The model under review builds one solid part; all positions refer to its coordinate system, in mm. A direction names the side the tool comes from. Give positions to 0.01 mm unless a question says otherwise; leave off trailing zeros. Order: outer loops, then holes, each group sorted by start corner. A loop starts at its lowest first (then second) coordinate and runs counter-clockwise, first axis right, second up. Notation, with made-up numbers: (79, 52) - (103, 52) arc R24 ccw to (103, 68) - close; hole circle Ø7 at (38.5, -29.75). An arc over 180 degrees is marked (long way). Write item = value, one per line. Start each with the question number.
1. Wall thickness on probe 1 along X at (y, z) = (62, 24) (3 decimals); probe 2 along X at (y, z) = (-233, 38.5); probe 3 along Y at (x, z) = (133, 7.5): over which ranges is each line inside the solid? List them lowest first.
2. Mouldability with a two-part tool opening along Y and no side actions: class faces 4 (the flat face through (322, 71.069, 70)), 5 (the flat face through (317.5, -165, 66)), 6 (the flat face through (176.452, 115.669, 10.908)) as pulls with the +Y half, pulls with the -Y half, needs draft (parallel to the pull), parting line crosses it, or undercut.
3. We need section B-B, the plane y = -259. Give the boundary of the cut face in (x, z) (3 decimals), and give its area (3 significant figures).
4. We need section C-C, the plane z = 73.5. Give the boundary of the cut face in (x, y) (3 decimals).
5. For P1, Ø7.5, axis at x = 320.5, z = 69, coming from the -Y side; P2, Ø6, axis at x = 322, z = 65.5, coming from the +Y side; P3, Ø6, axis at x = 162.5, z = 108.5, coming from the +Y side; P4, Ø3.5, axis at x = 147.5, y = 109, coming from the +Z side, all flat-tipped, find the tip position at first contact; note any pin that passes through.
6. We need section D-D, the plane y = -86. Give the boundary of the cut face in (x, z) (3 decimals), and give its area (3 significant figures).
7. We need section A-A, the plane x = 183. Give the boundary of the cut face in (y, z), and give its area (3 significant figures).
8. Machinability: for faces 1 (the flat face through (324, 74.244, 71)), 2 (the flat face through (0, -56, 50)), 3 (the flat face through (164.245, -284.866, 16.28)), which of the approach directions +Z, -Z, +X, -X, +Y, -Y give a long, thin tool a straight path to every point of the face, cutting with its end or side? Answer none if there is none.
from build123d import *

# Parameters (mm, degrees)
F1_DEPTH = 330
F2_T     = -3.175
F3_W     = 304.8
F3_H     = 101.6
F4_DEPTH = 254
F5_W     = 304.8
F5_H     = 254
F6_DEPTH = 25.4


with BuildPart() as f1:
    # F0 (on Right) → F1 (new body)
    with BuildSketch(Plane.YZ):
        Polygon((-18.4111015737, 126.7885861181), (-333.886384964, 0), (126.113615036, 0), (74.243833744, 54.1712634957), (74.243833744, 89.1712634957), align=None)
    extrude(amount=F1_DEPTH)

    # F2
    f2_openings = [f1.faces().sort_by_distance(p)[0] for p in [
        (165, -103.886385, 0),
    ]]
    offset(amount=F2_T, openings=f2_openings, kind=Kind.INTERSECTION)

    # F3 (on Front) → F4 (cut)
    with BuildSketch(Plane.XZ):
        with Locations((165.1896406174, 66.1754549101)):
            Rectangle(F3_W, F3_H)
    extrude(amount=-F4_DEPTH, mode=Mode.SUBTRACT)

    # F5 (on face) → F6 (cut)
    with BuildSketch(Plane(origin=(0, -46.4302683335, 115.5277656205), x_dir=(1, 0, 0), z_dir=(0, -0.3729076062, 0.9278684806))):
        with Locations((165.1, -127)):
            Rectangle(F5_W, F5_H)
    extrude(amount=-F6_DEPTH, mode=Mode.SUBTRACT)


solid = f1.part
Model answer:
q1.probe_1 = 0 to 3.175, 326.825 to 330
q1.probe_2 = 0 to 12.7, 317.5 to 330
q1.probe_3 = -315.22 to -306.71, 114.54 to 118.93
q2.face_4 = undercut
q2.face_5 = needs draft
q2.face_6 = pulls with the +Y half
q3.outline = (0, 0) - (3.175, 0) - (3.175, 26.675) - (12.7, 26.675) - (12.7, 30.097) - (0, 30.097) - close; (317.5, 26.675) - (326.825, 26.675) - (326.825, 0) - (330, 0) - (330, 30.097) - (317.5, 30.097) - close
q3.area = 256 mm2
q4.outline = (0, -151.004) - (12.7, -151.004) - (12.7, -142.49) - (3.175, -142.49) - (3.175, 71.069) - (12.79, 71.069) - (12.79, 74.244) - (0, 74.244) - close; (317.5, -151.004) - (330, -151.004) - (330, 74.244) - (317.59, 74.244) - (317.59, 71.069) - (326.825, 71.069) - (326.825, -142.49) - (317.5, -142.49) - close
q5.P1 = -171.53
q5.P2 = 74.24
q5.P3 = through
q5.P4 = 15.38
q6.outline = (0, 0) - (3.175, 0) - (3.175, 96.203) - (12.7, 96.203) - (12.7, 99.625) - (0, 99.625) - close; (317.5, 96.203) - (326.825, 96.203) - (326.825, 0) - (330, 0) - (330, 99.625) - (317.5, 99.625) - close
q6.area = 697 mm2
q7.outline = (-333.89, 0) - (-325.37, 0) - (-280.92, 17.86) - (-282.11, 20.81) - close; (-46.43, 115.53) - (-45.25, 112.58) - (-18.42, 123.36) - (0, 115.89) - (0, 116.98) - (5.76, 116.98) - (-18.41, 126.79) - close; (107, 15.38) - (121.72, 0) - (126.11, 0) - (111.39, 15.38) - close
q7.area = 396 mm2
q8.face_1 = +Z, +X, -X, +Y
q8.face_2 = +Z, -Z, -X, +Y, -Y
q8.face_3 = -Z
